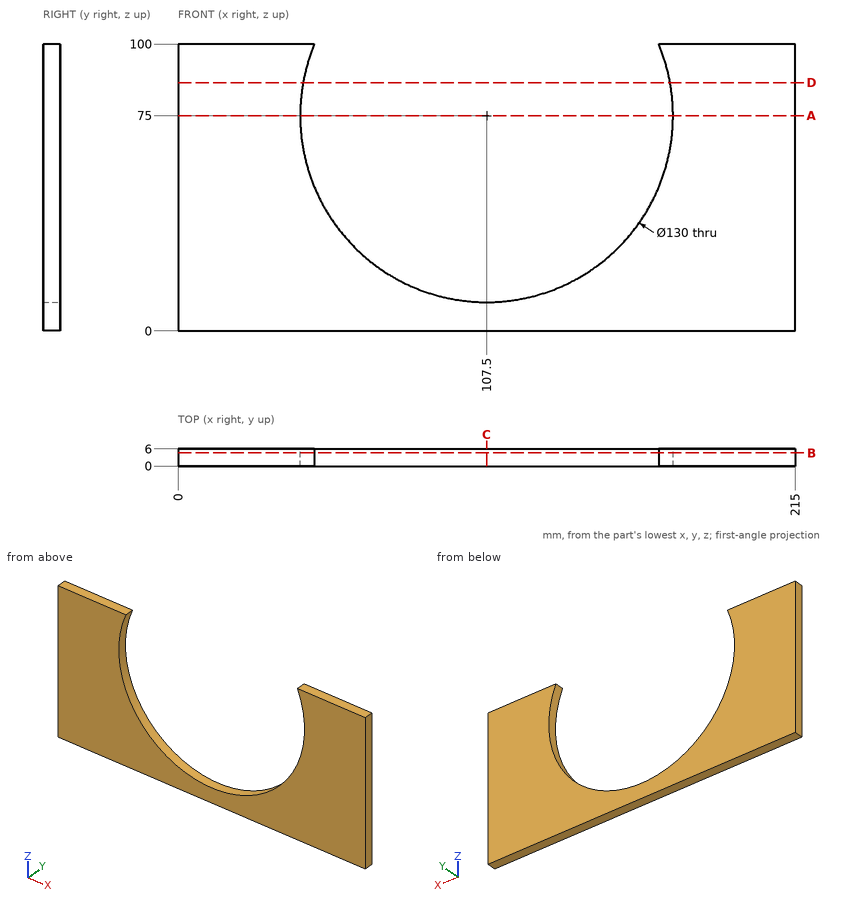
For this review, use the dimensioned drawing (mm, ordinates from the lowest corner) and the shaded views. Round coordinates to 2 decimals unless told otherwise and drop trailing zeros. Order: outer loops, then holes, each group sorted by start corner. A loop starts at its lowest first (then second) coordinate and runs counter-clockwise, first axis right, second up. Notation, with made-up numbers: M -8,5.5 L 12,5.5 A25 cw 12,24.5 Z; hole C -12,-0.75 d11. An arc over 180 degrees is marked long. Use a Markdown table: item, result. Add a question column.
Item 1: Add section B-B, the plane y = 4.6. Give the boundary of the cut face in (x, z), then the cut area to 3 significant figures.
Item 2: Add section C-C, the plane x = 107.5. Give the boundary of the cut face in (y, z), then the cut area to 3 significant figures.
Item 3: Add section A-A, the plane z = 75. Give the boundary of the cut face in (x, y), then the cut area to 3 significant figures.
Item 4: Add section D-D, the plane z = 86.5. Give the boundary of the cut face in (x, y), then the cut area to 3 significant figures.
Item 5: To check wall thickness, follow line 1 along X through (y, z) = (2.05, 75); line 2 along X through (y, z) = (5.3, 52); line 3 along Z through (x, y) = (109, 1.95). State the ranges of each line that lie inside material, in increasing order.
Geometry results:
| question | item | result |
|---|---|---|
| 1 | outline | M 0,0 L 215,0 L 215,100 L 167.5,100 A65 cw long 47.5,100 L 0,100 Z |
| 1 | area | 11,700 mm² |
| 2 | outline | M 0,0 L 6,0 L 6,10 L 0,10 Z |
| 2 | area | 60.0 mm² |
| 3 | outline | M 0,0 L 42.5,0 L 42.5,6 L 0,6 Z; M 172.5,0 L 215,0 L 215,6 L 172.5,6 Z |
| 3 | area | 510 mm² |
| 4 | outline | M 0,0 L 43.53,0 L 43.53,6 L 0,6 Z; M 171.47,0 L 215,0 L 215,6 L 171.47,6 Z |
| 4 | area | 522 mm² |
| 5 | line 1 | x = 0 to 42.5, 172.5 to 215 |
| 5 | line 2 | x = 0 to 46.71, 168.29 to 215 |
| 5 | line 3 | z = 0 to 10.02 |
